Input: part model. Units: mm. Frame: model coordinates. Round coordinates to 2 decimals unless told otherwise and drop trailing zeros. Loops run counter-clockwise (first coordinate to the right, second up) from the corner with the lowest first, then second, coordinate; pieces in that order, holes last.
(1) Cut plane D-D, the plane x = 40. Output: boundary loops of the cut face in (y, z).
(2) Cut plane C-C, the plane z = 5. Output: boundary loops of the cut face in (x, y), and give its area (3 significant figures).
(3) First-contact query: pin 1 Ø1.6 at (y, z) = (104, 5.5) entering from -X; pin 2 Ø2.5 at (x, z) = (104, 5.5) entering from -Y; pin 3 Ø6 at (y, z) = (70, 3) entering from +X. Flat tips, straight axial feed; report the tip coordinate or a pass-through.
(4) Cut plane B-B, the plane y = 40. Output: boundary loops of the cut face in (x, z).
(5) Line query: line 1 (Z direction, x = 12, y = 105); line 2 (Z direction, x = 105, y = 6.75); line 3 (Y direction, x = 5.75, z = 5). Output: solid intervals per line, ascending.
(6) Cut plane A-A, the plane x = 10. Output: boundary loops of the cut face in (y, z).
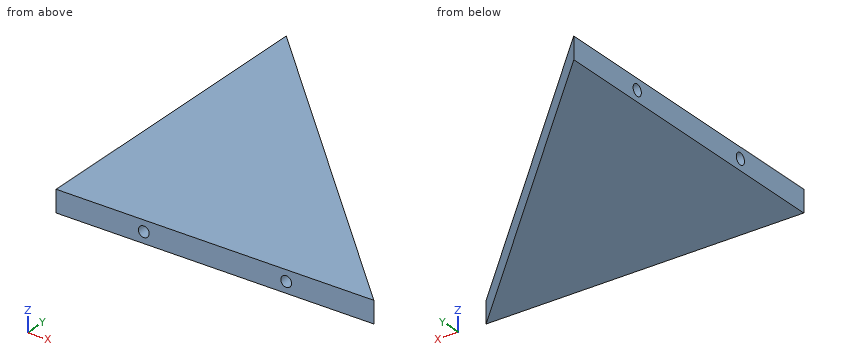
Autodesk Inventor part; units mm, degrees
ref_plane "YZ Plane" through (0, 0, 0) normal (1, 0, 0) x (0, 1, 0)
ref_plane "XZ Plane" through (0, 0, 0) normal (0, 1, 0) x (-1, 0, 0)
ref_plane "XY Plane" through (0, 0, 0) normal (0, 0, 1) x (1, 0, 0)
sketch "Sketch1" plane through (0, 0, 0) normal (0, 0, 1) x (1, 0, 0)
  line L0 (0, 0) -> (0, 145)
  line L1 (0, 145) -> (145, 0)
  line L2 (145, 0) -> (0, 0)
  dimension "d0" = 145
  dimension "d1" = 145
extrude "Extrusion1" add sketch "Sketch1" along normal blind 10
sketch "Sketch2" plane through (0, 0, 0) normal (0, -1, 0) x (1, 0, 0)
  line L0 (145, 0) -> (145, 10)
  line L1 (145, 5) -> (0, 5)
  circle A0 centre (105, 5) radius 3
  circle A1 centre (40, 5) radius 3
  line L2 (0, 0) -> (0, 10)
  dimension "d4" = 6
  dimension "d5" = 6
  dimension "d6" = 40
  dimension "d7" = 40
hole "Hole1" at (105, 0, 5) at (40, 0, 5) direction (0, 1, 0) diameter 4.917 depth 17.1
sketch "Sketch3" plane through (0, 0, 0) normal (-1, 0, 0) x (0, 0, 1)
  line L0 (0, 145) -> (10, 145)
  line L1 (5, 145) -> (5, 0)
  line L2 (0, 0) -> (10, 0)
  circle A0 centre (5, 105) radius 3
  circle A1 centre (5, 40) radius 3
  dimension "d15" = 6
  dimension "d16" = 6
  dimension "d17" = 40
  dimension "d18" = 40
hole "Hole2" at (0, 105, 5) at (0, 40, 5) direction (1, 0, 0) diameter 5.1881 depth 17.1
sketch "Sketch4" plane through (0, 0, 0) normal (-1, 0, 0) x (0, 0, 1)
  point P0 (0, 0)
properties part number "145x145(li)"
Reported:
1. outline: (0, 0) - (105, 0) - (105, 10) - (0, 10) - (0, 7.46) - (17.1, 7.46) - (17.1, 2.54) - (0, 2.54) - close
2. outline: (0, 0) - (37.54, 0) - (37.54, 17.1) - (42.46, 17.1) - (42.46, 0) - (102.54, 0) - (102.54, 17.1) - (107.46, 17.1) - (107.46, 0) - (145, 0) - (0, 145) - (0, 107.59) - (17.1, 107.59) - (17.1, 102.41) - (0, 102.41) - (0, 42.59) - (17.1, 42.59) - (17.1, 37.41) - (0, 37.41) - close
2. area: 10,200 mm2
3. pin 1: stops at x = 17.1
3. pin 2: stops at y = 17.1
3. pin 3: stops at x = 78
4. outline: (0, 0) - (105, 0) - (105, 10) - (0, 10) - (0, 7.59) - (17.1, 7.59) - (17.1, 2.41) - (0, 2.41) - close
5. line 1: z = 0 to 2.41, 7.59 to 10
5. line 2: z = 0 to 2.54, 7.46 to 10
5. line 3: y = 0 to 37.41, 42.59 to 102.41, 107.59 to 139.25
6. outline: (0, 0) - (135, 0) - (135, 10) - (0, 10) - close; hole circle Ø5.19 at (40, 5); hole circle Ø5.19 at (105, 5)
